Work out the finished part from the listing and answer in its coordinate system (mm). A direction names the side the tool comes from. Give positions to 0.01 mm unless a question says otherwise; leave off trailing zeros. Write each loop counter-clockwise with the first axis right and the second up, starting at its lowest first coordinate (ties: lowest second). Pieces come first, ordered by that corner, then holes. Notation, with made-up numbers: (45, 49) - (64, 49) arc R18 cw to (64, 76) - close; hole circle Ø11 at (-10, 18.25). An arc over 180 degrees is marked (long way). Write item = value, one per line.
from build123d import *

# Parameters (mm, degrees)
F0_W         = 70
F0_H         = 70
F1_DEPTH     = 40
F3_DEPTH     = 78
F4_W         = 25
F4_H         = 17.3788098246
F5_DEPTH     = 72.2
F6_T1_DEPTH  = 70
F6_T3_DEPTH  = 40
F6_T5_DEPTH  = 65
F6_T7_DEPTH  = 37.5
F6_T9_DEPTH  = 95
F6_T12_ANGLE = 90
F6_T14_ANGLE = 90
F6_T16_ANGLE = 90
F6_T18_ANGLE = 90


# Not quite as in the source:
# - a fillet or chamfer that OpenCascade refuses, or shapes differently, is made with other operations: its cross-section is extruded or revolved along the edge and cut away or added
# - a feature names something its author has since deleted; it is built from what else it names


with BuildPart() as f1:
    # F0 (on Top) → F1 (new body)
    with BuildSketch(Plane.XY):
        Rectangle(F0_W, F0_H)
    extrude(amount=F1_DEPTH)

    # F2 (on face) → F3 (cut)
    with BuildSketch(Plane.XZ.offset(35)):
        with BuildLine():
            ThreePointArc((29.5, 27.4665858597), (21.5, 35.4665858597), (13.5, 27.4665858597))
            ThreePointArc((13.5, 27.4665858597), (21.5, 19.4665858597), (29.5, 27.4665858597))
        make_face()
        with BuildLine():
            ThreePointArc((8, 27.4665858597), (0, 35.4665858597), (-8, 27.4665858597))
            ThreePointArc((-8, 27.4665858597), (0, 19.4665858597), (8, 27.4665858597))
        make_face()
        with BuildLine():
            ThreePointArc((-13.5, 27.4665858597), (-21.5, 35.4665858597), (-29.5, 27.4665858597))
            ThreePointArc((-29.5, 27.4665858597), (-21.5, 19.4665858597), (-13.5, 27.4665858597))
        make_face()
    extrude(amount=-F3_DEPTH, mode=Mode.SUBTRACT)

    # F4 (on face) → F5 (cut)
    with BuildSketch(Plane(origin=(-35, 0, 0), x_dir=(0, -1, 0), z_dir=(-1, 0, 0))):
        with Locations((-12.5, 31.3105950877)):
            Rectangle(F4_W, F4_H)
        with Locations((12.5, 31.3105950877)):
            Rectangle(F4_W, F4_H)
        Polygon((25, 22.6211901754), (0, 22.6211901754), (-25, 22.6211901754), (-25, 10), (25, 10), align=None)
    extrude(amount=-F5_DEPTH, mode=Mode.SUBTRACT)

    # F6: fillet of radius 5 on 16 edges, made by hand

    # F6_s2 → F6_t1 (join)
    with BuildSketch(Plane.YZ.offset(-35)):
        with BuildLine():
            ThreePointArc((20, 10), (23.5355339059, 11.4644660941), (25, 15))
            Line((25, 15), (25, 10))
            Line((25, 10), (20, 10))
        make_face()
        with BuildLine():
            ThreePointArc((-25, 15), (-23.5355339059, 11.4644660941), (-20, 10))
            Line((-20, 10), (-25, 10))
            Line((-25, 10), (-25, 15))
        make_face()
    extrude(amount=F6_T1_DEPTH)

    # F6_s4 → F6_t3 (cut)
    with BuildSketch(Plane.XZ.offset(-20)):
        with BuildLine():
            ThreePointArc((35, 5), (33.5355339059, 8.5355339059), (30, 10))
            Line((30, 10), (35, 10))
            Line((35, 10), (35, 5))
        make_face()
        with BuildLine():
            ThreePointArc((-35, 5), (-33.5355339059, 8.5355339059), (-30, 10))
            Line((-30, 10), (-35, 10))
            Line((-35, 10), (-35, 5))
        make_face()
    extrude(amount=F6_T3_DEPTH, mode=Mode.SUBTRACT)

    # F6_s6 → F6_t5 (cut)
    with BuildSketch(Plane.XY.offset(-12.5)):
        with BuildLine():
            ThreePointArc((30, -35), (33.5355339059, -33.5355339059), (35, -30))
            Line((35, -30), (35, -35))
            Line((35, -35), (30, -35))
        make_face()
        with BuildLine():
            ThreePointArc((35, 30), (33.5355339059, 33.5355339059), (30, 35))
            Line((30, 35), (35, 35))
            Line((35, 35), (35, 30))
        make_face()
        with BuildLine():
            ThreePointArc((-35, 30), (-33.5355339059, 33.5355339059), (-30, 35))
            Line((-30, 35), (-35, 35))
            Line((-35, 35), (-35, 30))
        make_face()
        with BuildLine():
            ThreePointArc((-30, -35), (-33.5355339059, -33.5355339059), (-35, -30))
            Line((-35, -30), (-35, -35))
            Line((-35, -35), (-30, -35))
        make_face()
    extrude(amount=F6_T5_DEPTH, mode=Mode.SUBTRACT)

    # F6_s8 → F6_t7 (cut)
    with BuildSketch(Plane.XY.offset(15)):
        with BuildLine():
            ThreePointArc((-35, 30), (-33.5355339059, 26.4644660941), (-30, 25))
            Line((-30, 25), (-35, 25))
            Line((-35, 25), (-35, 30))
        make_face()
        with BuildLine():
            ThreePointArc((-35, -30), (-33.5355339059, -26.4644660941), (-30, -25))
            Line((-30, -25), (-35, -25))
            Line((-35, -25), (-35, -30))
        make_face()
        with BuildLine():
            ThreePointArc((35, 30), (33.5355339059, 26.4644660941), (30, 25))
            Line((30, 25), (35, 25))
            Line((35, 25), (35, 30))
        make_face()
        with BuildLine():
            ThreePointArc((35, -30), (33.5355339059, -26.4644660941), (30, -25))
            Line((30, -25), (35, -25))
            Line((35, -25), (35, -30))
        make_face()
    extrude(amount=F6_T7_DEPTH, mode=Mode.SUBTRACT)

    # F6_s10 → F6_t9 (cut)
    with BuildSketch(Plane.YZ.offset(-47.5)):
        with BuildLine():
            ThreePointArc((-30, 40), (-26.4644660941, 38.5355339059), (-25, 35))
            Line((-25, 35), (-25, 40))
            Line((-25, 40), (-30, 40))
        make_face()
        with BuildLine():
            ThreePointArc((-35, 35), (-33.5355339059, 38.5355339059), (-30, 40))
            Line((-30, 40), (-35, 40))
            Line((-35, 40), (-35, 35))
        make_face()
        with BuildLine():
            ThreePointArc((30, 40), (33.5355339059, 38.5355339059), (35, 35))
            Line((35, 35), (35, 40))
            Line((35, 40), (30, 40))
        make_face()
        with BuildLine():
            ThreePointArc((25, 35), (26.4644660941, 38.5355339059), (30, 40))
            Line((30, 40), (25, 40))
            Line((25, 40), (25, 35))
        make_face()
    extrude(amount=F6_T9_DEPTH, mode=Mode.SUBTRACT)

    # F6_s11 → F6_t12 (revolve, cut)
    with BuildSketch(Plane.XY.offset(15)):
        with BuildLine():
            ThreePointArc((35, -30), (33.5355339059, -26.4644660941), (30, -25))
            Line((30, -25), (35, -25))
            Line((35, -25), (35, -30))
        make_face()
    revolve(axis=Axis((35, -20, 15), (1, 0, 0)), revolution_arc=F6_T12_ANGLE, mode=Mode.SUBTRACT)

    # F6_s13 → F6_t14 (revolve, cut)
    with BuildSketch(Plane.XZ.offset(-20)):
        with BuildLine():
            ThreePointArc((35, 5), (33.5355339059, 8.5355339059), (30, 10))
            Line((30, 10), (35, 10))
            Line((35, 10), (35, 5))
        make_face()
    revolve(axis=Axis((35, 20, 15), (1, 0, 0)), revolution_arc=F6_T14_ANGLE, mode=Mode.SUBTRACT)

    # F6_s15 → F6_t16 (revolve, cut)
    with BuildSketch(Plane.XZ.offset(-20)):
        with BuildLine():
            ThreePointArc((-35, 5), (-33.5355339059, 8.5355339059), (-30, 10))
            Line((-30, 10), (-35, 10))
            Line((-35, 10), (-35, 5))
        make_face()
    revolve(axis=Axis((-35, 20, 15), (1, 0, 0)), revolution_arc=F6_T16_ANGLE, mode=Mode.SUBTRACT)

    # F6_s17 → F6_t18 (revolve, cut)
    with BuildSketch(Plane.XY.offset(15)):
        with BuildLine():
            ThreePointArc((-35, -30), (-33.5355339059, -26.4644660941), (-30, -25))
            Line((-30, -25), (-35, -25))
            Line((-35, -25), (-35, -30))
        make_face()
    revolve(axis=Axis((-35, -20, 15), (1, 0, 0)), revolution_arc=F6_T18_ANGLE, mode=Mode.SUBTRACT)


solid = f1.part
1. Find section C-C, the plane x = -11.5. Give the vertices of the cut face in (y, z), then the cut area to 3 significant figures.
Solution:
outline = (-35, 0) - (35, 0) - (35, 35) arc R5 ccw to (25, 35) - (25, 15) arc R5 cw to (20, 10) - (-20, 10) arc R5 cw to (-25, 15) - (-25, 35) arc R5 ccw to (-35, 35) - close
area = 1,290 mm^2
2. Find section B-B, the plane x = -21. Give the vertices of the cut face in (y, z), then the cut area to 3 significant figures.
Solution:
outline = (-35, 0) - (35, 0) - (35, 19.48) - (25, 19.48) - (25, 15) arc R5 cw to (20, 10) - (-20, 10) arc R5 cw to (-25, 15) - (-25, 19.48) - (-35, 19.48) - close; (-34.98, 35.45) - (-25.02, 35.45) arc R5 ccw to start; (25.02, 35.45) - (34.98, 35.45) arc R5 ccw to start
area = 970 mm^2
3. A tool of negligible diameter and unlimited length cuts with its end or side. For faces 1 (the cylindrical face through (0, -24, 12)), 2 (the cylindrical face through (-34, 0, 8)), 3 (the cylindrical face through (1.041, 29.93, 19.535)), 4 (the flat face through (-35, 0, 3)), 5 (the cylindrical face through (34, 0, 8)), from which of +Z, -Z, +X, -X, +Y, -Y can it reach the whole face along a straight path? Write none if from no direction.
Solution:
face_1 = +Z, +X, -X
face_2 = +Z, -X
face_3 = +Y, -Y
face_4 = +Z, -Z, -X, +Y, -Y
face_5 = +Z, +X
4. Find section D-D, the plane y = 2.5. Give the vertices of the cut face in (x, z).
Solution:
outline = (-35, 0) - (35, 0) - (35, 5) arc R5 ccw to (30, 10) - (-30, 10) arc R5 ccw to (-35, 5) - close
5. Given pin 1 (12 mm diameter, centred on x = -5, y = -3.5, fed in from +Z); pin 2 (13 mm diameter, centred on x = -21.5, z = 27.47, fed in from +Y); pin 3 (8 mm diameter, centred on y = 14, z = 11, fed in from -X), each flat-ended and moving along its own axis, determine where each tip first touches the part or whether it passes through.
Solution:
pin_1 = 10
pin_2 = through
pin_3 = -34.58
6. Straight lines are drawn through the part: line 1 (Y direction, x = 12, z = 15.5); line 2 (X direction, y = -31.5, z = 30); line 3 (Z direction, x = -30, y = 9). For each, find the intervals that lie inside material, in ascending order.
Solution:
line_1 = -35 to -25, 25 to 35
line_2 = -34.77 to -29.09, -13.91 to -7.59, 7.59 to 13.91, 29.09 to 34.77
line_3 = 0 to 10
7. Find section A-A, the plane z = 17.5. Give the vertices of the cut face in (x, y).
Solution:
outline = (-30, -35) - (30, -35) arc R5 ccw to (30, -25) - (-30, -25) arc R5 ccw to start; (-30, 25) - (30, 25) arc R5 ccw to (30, 35) - (-30, 35) arc R5 ccw to start
8. For a pull along Y with two mould halves and no side action, classify faces 6 (the flat face through (0, 35, 13)), 7 (the cylindrical face through (29.492, -30.07, 27.115)), 8 (the cylindrical face through (0, 23, 11)) as pulls with the +Y half, pulls with the -Y half, needs draft (parallel to the pull), parting line crosses it, or undercut.
Solution:
face_6 = pulls with the +Y half
face_7 = needs draft
face_8 = undercut
